Design review of the part built by this model. Coordinates are the model's own, in mm. A direction names the side the tool comes from. Give positions to 0.01 mm unless a question says otherwise; leave off trailing zeros. Order: outer loops, then holes, each group sorted by start corner. A loop starts at its lowest first (then second) coordinate and runs counter-clockwise, first axis right, second up. Notation, with made-up numbers: (-12.5, -35.5) - (3.5, -35.5) arc R27 cw to (3.5, -11.5) - close; hole circle Ø9 at (75.25, -22.75). An arc over 180 degrees is marked (long way). Write each question's results on one line, items separated by ' | '. Start each with the question number.
```python
from build123d import *

# Parameters (mm, degrees)
EXTRUDE_4_DEPTH             = 1
EXTRUDE_5_DEPTH             = 19
SKETCH_12_R                 = 0.8
EXTRUDE_7_DEPTH             = 8
SKETCH_13_R                 = 0.5
CUT_EXTRUDE_1_DEPTH         = 3
PATTERN_LINEAR_1_COUNT      = 2
PATTERN_LINEAR_1_PITCH      = 44
PATTERN_LINEAR_1_COUNT_DIR2 = 2
PATTERN_LINEAR_1_PITCH_DIR2 = 44
PATTERN_LINEAR_2_COUNT      = 2
PATTERN_LINEAR_2_PITCH      = 44
PATTERN_LINEAR_2_COUNT_DIR2 = 2
PATTERN_LINEAR_2_PITCH_DIR2 = 44


with BuildPart() as part:
    # 草图1 → 凸台-拉伸4 (new body)
    with BuildSketch(Plane.XY):
        with BuildLine():
            Line((22, 25), (-22, 25))
            ThreePointArc((-22, 25), (-24.121320344, 24.121320344), (-25, 22))
            Line((-25, 22), (-25, -22))
            ThreePointArc((-25, -22), (-24.121320344, -24.121320344), (-22, -25))
            Line((-22, -25), (22, -25))
            ThreePointArc((22, -25), (24.121320344, -24.121320344), (25, -22))
            Line((25, -22), (25, 22))
            ThreePointArc((25, 22), (24.121320344, 24.121320344), (22, 25))
        make_face()
    extrude(amount=EXTRUDE_4_DEPTH)

    # 草图7 → 凸台-拉伸5 (add)
    with BuildSketch(Plane.XY.offset(1)):
        with BuildLine():
            ThreePointArc((22, -25), (24.121320344, -24.121320344), (25, -22))
            Line((25, -22), (25, 22))
            ThreePointArc((25, 22), (24.121320344, 24.121320344), (22, 25))
            Line((22, 25), (-22, 25))
            ThreePointArc((-22, 25), (-24.121320344, 24.121320344), (-25, 22))
            Line((-25, 22), (-25, -22))
            ThreePointArc((-25, -22), (-24.121320344, -24.121320344), (-22, -25))
            Line((-22, -25), (22, -25))
        make_face()
        with BuildLine():
            Line((22, -24), (-22, -24))
            ThreePointArc((-22, -24), (-23.414213562, -23.414213562), (-24, -22))
            Line((-24, -22), (-24, 22))
            ThreePointArc((-24, 22), (-23.414213562, 23.414213562), (-22, 24))
            Line((-22, 24), (22, 24))
            ThreePointArc((22, 24), (23.414213562, 23.414213562), (24, 22))
            Line((24, 22), (24, -22))
            ThreePointArc((24, -22), (23.414213562, -23.414213562), (22, -24))
        make_face(mode=Mode.SUBTRACT)
    extrude(amount=EXTRUDE_5_DEPTH)

    # 草图12 → 凸台-拉伸7 (add)
    with BuildSketch(Plane.XY.offset(1)):
        with Locations((-22, 22)):
            Circle(SKETCH_12_R)
    extrude_7 = extrude(amount=EXTRUDE_7_DEPTH)

    # 草图13 → 切除-拉伸1 (cut)
    with BuildSketch(Plane.XY.offset(9)):
        with Locations((-22, 22)):
            Circle(SKETCH_13_R)
    cut_extrude_1 = extrude(amount=-CUT_EXTRUDE_1_DEPTH, mode=Mode.SUBTRACT)

    # 阵列(线性)1: Extrude 7 2 × 2
    with Locations(*[(i * PATTERN_LINEAR_1_PITCH, -j * PATTERN_LINEAR_1_PITCH_DIR2, 0) for i in range(PATTERN_LINEAR_1_COUNT) for j in range(PATTERN_LINEAR_1_COUNT_DIR2) if (i, j) != (0, 0)]):
        add(extrude_7)

    # 阵列(线性)2: Cut-Extrude 1 2 × 2
    with Locations(*[Vector(1, 0, 0) * (i * PATTERN_LINEAR_2_PITCH) + Vector(1, 0, 0) * (j * PATTERN_LINEAR_2_PITCH_DIR2) for i in range(PATTERN_LINEAR_2_COUNT) for j in range(PATTERN_LINEAR_2_COUNT_DIR2) if (i, j) != (0, 0)]):
        add(cut_extrude_1, mode=Mode.SUBTRACT)


solid = part.part
```
Q1. Add section C-C (z = 14.25). Give the boundary of the cut face in (x, y).
Q2. Draft analysis for pull direction Y (two halves, no side actions). For faces 3 (the flat face through (-24.2, 11.2, 20)), 4 (the cylindrical face through (24.1, -24.14, 9.86)), 5 (the flat face through (22, -22, 9)), 6 (the flat face through (0, -24, 10)), state which applies: pulls with the +Y half, pulls with the -Y half, needs draft (parallel to the pull), parting line crosses it, or undercut.
Q3. Insertion check: pin 1 Ø4 at (x, y) = (16.5, -9) entering from -Z; pin 2 Ø0.8 at (x, y) = (-21.5, 22) entering from +Z; pin 3 Ø0.8 at (x, y) = (-22, 22) entering from +Z; pin 4 Ø24 at (x, y) = (-4.5, 1) entering from +Z. Each pin has a flat end and moves straight along its axis. Give the tip position at first contact, or say it passes through.
Q4. Add section B-B (x = -16.5). Give the boundary of the cut face in (y, z), plus the area to 3 significant figures.
Q5. For line 1 (Y direction, x = 22, z = 7.1); line 2 (Y direction, x = 10, z = 2.25), list the stretches that pass through material, from the lowest coordinate up. Write a range as [from, to].
Q6. Add section A-A (z = 7.25). Give the boundary of the cut face in (x, y).
Q7. Machinability: for faces 1 (the flat face through (24, 0, 10)), 2 (the cylindrical face through (-24.14, -24.1, 9.86)), which of the approach directions +Z, -Z, +X, -X, +Y, -Y give a long, thin tool a straight path to every point of the face, cutting with its end or side? Answer none if there is none.
Verdict:
1) outline: (-25, -22) arc R3 ccw to (-22, -25) - (22, -25) arc R3 ccw to (25, -22) - (25, 22) arc R3 ccw to (22, 25) - (-22, 25) arc R3 ccw to (-25, 22) - close; hole (-24, -22) arc R2 ccw to (-22, -24) - (22, -24) arc R2 ccw to (24, -22) - (24, 22) arc R2 ccw to (22, 24) - (-22, 24) arc R2 ccw to (-24, 22) - close
2) face 3: needs draft | face 4: pulls with the -Y half | face 5: undercut | face 6: undercut
3) pin 1: stops at z = 0 | pin 2: stops at z = 9 | pin 3: stops at z = 6 | pin 4: stops at z = 1
4) outline: (-25, 0) - (25, 0) - (25, 20) - (24, 20) - (24, 1) - (-24, 1) - (-24, 20) - (-25, 20) - close | area: 88.0 mm2
5) line 1: y = [-25, -24], [-22.8, -21.2], [21.2, 21.5], [22.5, 22.8], [24, 25] | line 2: y = [-25, -24], [24, 25]
6) outline: (-25, -22) arc R3 ccw to (-22, -25) - (22, -25) arc R3 ccw to (25, -22) - (25, 22) arc R3 ccw to (22, 25) - (-22, 25) arc R3 ccw to (-25, 22) - close; circle Ø1.6 at (-22, -22); circle Ø1.6 at (-22, 22); circle Ø1.6 at (22, -22); circle Ø1.6 at (22, 22); hole (-24, -22) arc R2 ccw to (-22, -24) - (22, -24) arc R2 ccw to (24, -22) - (24, 22) arc R2 ccw to (22, 24) - (-22, 24) arc R2 ccw to (-24, 22) - close; hole circle Ø1 at (-22, 22); hole circle Ø1 at (22, 22)
7) face 1: +Z | face 2: +Z, -Z, -X, -Y
